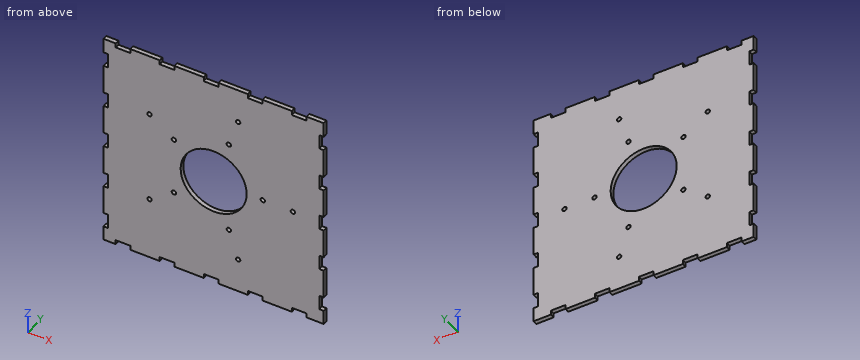
from build123d import *

# Parameters (mm, degrees)
SKETCH1_W           = 150
SKETCH1_H           = 150
BOSS_EXTRUDE1_DEPTH = 3
SKETCH2_R           = 22.5
CUT_EXTRUDE1_DEPTH  = 3
SKETCH3_W           = 10
SKETCH3_H           = 3
CUT_EXTRUDE2_DEPTH  = 3
LPATTERN1_COUNT     = 5
LPATTERN1_PITCH     = 30
SKETCH4_W           = 3
SKETCH4_H           = 10
CUT_EXTRUDE3_DEPTH  = 3
LPATTERN2_COUNT     = 5
LPATTERN2_PITCH     = 30
SKETCH5_R           = 1.5
CUT_EXTRUDE4_DEPTH  = 10


with BuildPart() as part:
    # Sketch1 → Boss-Extrude1 (new body)
    with BuildSketch(Plane(origin=(0, 0, 0), x_dir=(-1, 0, 0), z_dir=(0, 1, 0))):
        Rectangle(SKETCH1_W, SKETCH1_H)
    extrude(amount=BOSS_EXTRUDE1_DEPTH)

    # Sketch2 → Cut-Extrude1 (cut)
    with BuildSketch(Plane(origin=(0, 3, 0), x_dir=(1, 0, 0), z_dir=(0, 1, 0))):
        with Locations(Location((0, 0, 0), (0, 0, 270))):
            Circle(SKETCH2_R)
    extrude(amount=-CUT_EXTRUDE1_DEPTH, mode=Mode.SUBTRACT)

    # Sketch3 → Cut-Extrude2 (cut)
    with BuildSketch(Plane(origin=(0, 3, 0), x_dir=(1, 0, 0), z_dir=(0, 1, 0))):
        with Locations((-61.749963879, 73.5)):
            Rectangle(SKETCH3_W, SKETCH3_H)
        with Locations((-61.749963879, -73.5)):
            Rectangle(SKETCH3_W, SKETCH3_H)
    cut_extrude2 = extrude(amount=-CUT_EXTRUDE2_DEPTH, mode=Mode.SUBTRACT)

    # LPattern1: Cut-Extrude2 ×5
    with Locations(*[(i * LPATTERN1_PITCH, 0, 0) for i in range(1, LPATTERN1_COUNT)]):
        add(cut_extrude2, mode=Mode.SUBTRACT)

    # Sketch4 → Cut-Extrude3 (cut)
    with BuildSketch(Plane(origin=(0, 3, 0), x_dir=(1, 0, 0), z_dir=(0, 1, 0))):
        with Locations((-73.5, -59.825317059)):
            Rectangle(SKETCH4_W, SKETCH4_H)
        with Locations((73.5, -59.825317059)):
            Rectangle(SKETCH4_W, SKETCH4_H)
    cut_extrude3 = extrude(amount=-CUT_EXTRUDE3_DEPTH, mode=Mode.SUBTRACT)

    # LPattern2: Cut-Extrude3 ×5
    with Locations(*[(0, 0, -i * LPATTERN2_PITCH) for i in range(1, LPATTERN2_COUNT)]):
        add(cut_extrude3, mode=Mode.SUBTRACT)

    # Sketch5 → Cut-Extrude4 (cut)
    with BuildSketch(Plane(origin=(0, 0, 0), x_dir=(-1, 0, 0), z_dir=(0, -1, 0))):
        with Locations(Location((-33.5, 0, 0), (0, 0, 180))):
            Circle(SKETCH5_R)
        with Locations(Location((-10.352069312, 31.860393296, 0), (0, 0, 180))):
            Circle(SKETCH5_R)
        with Locations(Location((27.102069312, 19.690805952, 0), (0, 0, 180))):
            Circle(SKETCH5_R)
        with Locations(Location((27.102069312, -19.690805952, 0), (0, 0, 180))):
            Circle(SKETCH5_R)
        with Locations(Location((-10.352069312, -31.860393296, 0), (0, 0, 180))):
            Circle(SKETCH5_R)
        with Locations(Location((-54, 0, 0), (0, 0, 180))):
            Circle(SKETCH5_R)
        with Locations(Location((-16.686917696, 51.35705188, 0), (0, 0, 180))):
            Circle(SKETCH5_R)
        with Locations(Location((43.686917696, 31.740403624, 0), (0, 0, 180))):
            Circle(SKETCH5_R)
        with Locations(Location((43.686917696, -31.740403624, 0), (0, 0, 180))):
            Circle(SKETCH5_R)
        with Locations(Location((-16.686917696, -51.35705188, 0), (0, 0, 180))):
            Circle(SKETCH5_R)
    extrude(amount=-CUT_EXTRUDE4_DEPTH, mode=Mode.SUBTRACT)


solid = part.part
The model under review builds one solid part; all positions refer to its coordinate system, in mm. Round coordinates to 2 decimals unless told otherwise and drop trailing zeros. Loops run counter-clockwise (first coordinate to the right, second up) from the corner with the lowest first, then second, coordinate; pieces in that order, holes last. Notation, with made-up numbers: (-37.75, 71.25) -> (-0.75, 71.25) arc R24 ccw to (-0.75, 91.25) -> close; hole circle Ø10 at (80.5, -31.5). An arc over 180 degrees is marked (long way). Write item = value, one per line. Start each with the question number.
Item 1: Take a section at A-A on x = 0. Give the boundary of the cut face in (y, z), plus the area to 3 significant figures.
Item 2: Insertion check: pin 1 (0.9 mm diameter, centred on y = 1, z = 29, fed in from +X); pin 2 (2.5 mm diameter, centred on x = 10.35, z = -31.86, fed in from +Y); pin 3 (0.9 mm diameter, centred on x = 26.5, y = 1.5, fed in from -Z). Each pin has a flat end and moves straight along its axis. Give the tip position at first contact, or say it passes through.
Item 3: Take a section at D-D on y = 1.05. Count the separate pieces of the cut face and the enclosed holes in it, plus the area to 3 significant figures.
Item 4: Take a section at C-C on z = -27. Give the boundary of the cut face in (x, y).
Item 5: To check wall thickness, follow L1, parallel to Z at x = 15.5, y = 1; L2, parallel to Z at x = -34.5, y = 2.3. State the ranges of each line that lie inside material, in increasing order.
Item 6: Take a section at B-B on z = 16. Give the boundary of the cut face in (x, y).
Result:
q1.outline = (0, -72) -> (3, -72) -> (3, -22.5) -> (0, -22.5) -> close; (0, 22.5) -> (3, 22.5) -> (3, 72) -> (0, 72) -> close
q1.area = 297 mm²
q2.pin_1 = 72
q2.pin_2 = through
q2.pin_3 = -72
q3.separate_pieces = 1
q3.enclosed_holes = 11
q3.area = 20,200 mm²
q4.outline = (-72, 0) -> (72, 0) -> (72, 3) -> (-72, 3) -> close
q5.L1 = -75 to -52.27, -50.44 to -16.31, 16.31 to 50.44, 52.27 to 75
q5.L2 = -72 to 72
q6.outline = (-75, 0) -> (-15.82, 0) -> (-15.82, 3) -> (-75, 3) -> close; (15.82, 0) -> (75, 0) -> (75, 3) -> (15.82, 3) -> close
